The drawing under review shows one solid part. Ordinate dimensions are in mm from its lowest x, y, z. Give positions to 0.01 mm unless a question says otherwise; leave off trailing zeros. Loops run counter-clockwise (first coordinate to the right, second up) from the corner with the lowest first, then second, coordinate; pieces in that order, holes last. Notation, with made-up numbers: M 2.5,28.5 L 60.5,28.5 A15 cw 60.5,57.5 Z; hole C -3.75,18.25 d2. An arc over 180 degrees is marked long. Put each result on its own line as item: value. Start each with the question number.
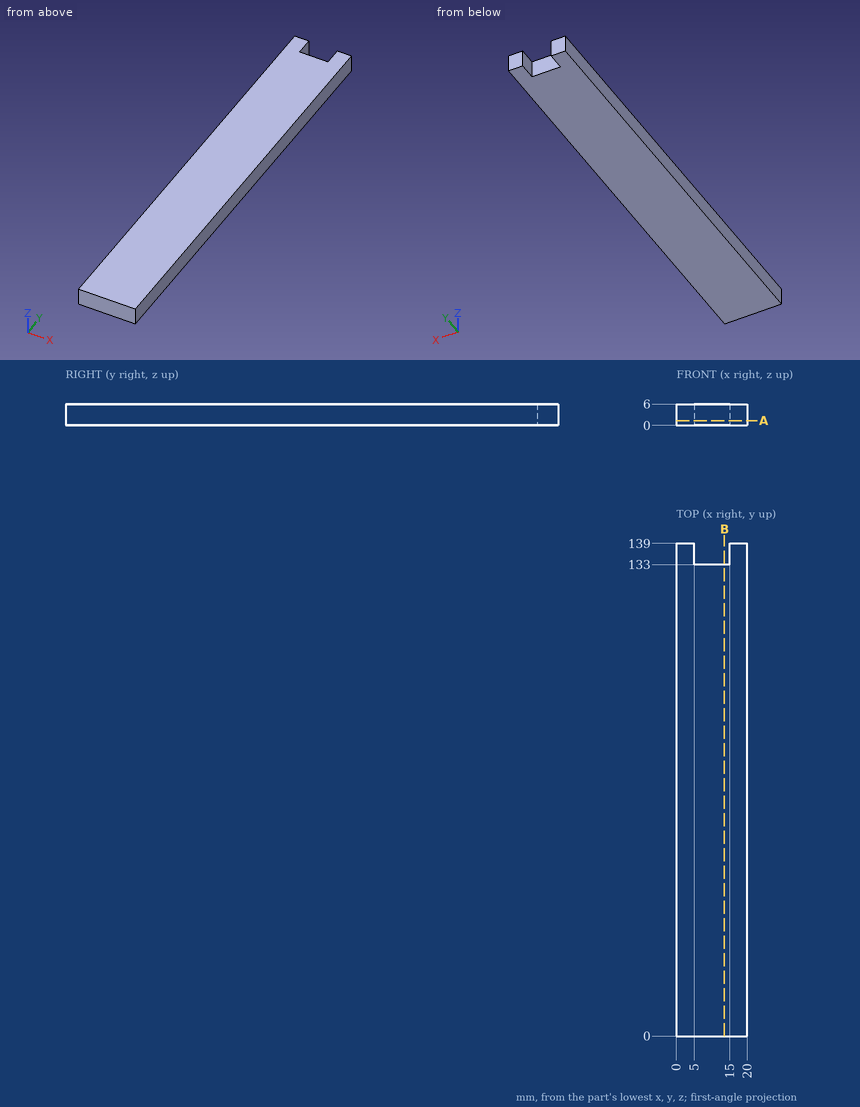
(1) To check wall thickness, follow L1, parallel to Y at x = 6, z = 4.15. State the ranges of the line that lie inside material, in increasing order. Write a range as [from, to].
(2) Insertion check: pin 1 (3 mm diameter, centred on x = 12.5, z = 3.5, fed in from +Y). The pin has a flat end and moves straight along its axis. Give the tip position at first contact, or say it passes through.
(3) We need section A-A, the plane z = 1.3. Write out the cut boundary in (x, y), plus the area to 3 significant figures.
(4) We need section B-B, the plane x = 13.5. Write out the cut boundary in (y, z), plus the area to 3 significant figures.
Check sheet entries:
1. L1: y = [0, 133]
2. pin 1: stops at y = 133
3. outline: M 0,0 L 20,0 L 20,139 L 15,139 L 15,133 L 5,133 L 5,139 L 0,139 Z
3. area: 2,720 mm²
4. outline: M 0,0 L 133,0 L 133,6 L 0,6 Z
4. area: 798 mm²
